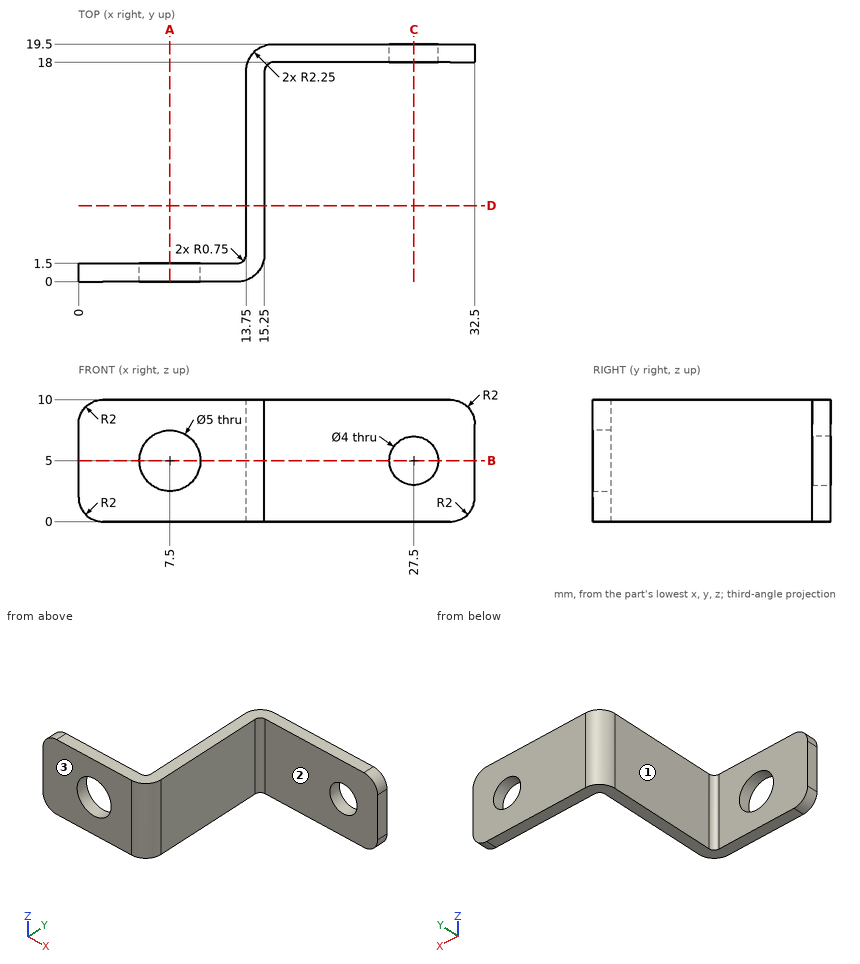
Geometry: see drawing. Coordinates: mm, zero at the bounding-box minimum. A direction names the side the tool comes from. Give positions to 0.01 mm unless a question says otherwise; leave off trailing zeros. Loops run counter-clockwise (first coordinate to the right, second up) from the corner with the lowest first, then second, coordinate; pieces in that order, holes last. Notation, with made-up numbers: (51, 88.25) - (91, 88.25) arc R23 cw to (91, 122.25) - close; hole circle Ø5 at (4.25, -37). An arc over 180 degrees is marked (long way). Use CSV: the item, a comma, the result in double quotes. Start each with the question number.
Item 1: Section B-B on z = 5. Return loops of the section in (x, y), then the cut area to 3 significant figures.
Item 2: Contact query for flat-ended pins moving along their axis: P1, Ø5, axis at y = 12, z = 9, coming from the +X side; P2, Ø4, axis at y = 10, z = 2, coming from the -X side; P3, Ø5, axis at x = 27, z = 4.5, coming from the -Y side. Output: stop coordinate, or through.
Item 3: Section A-A on x = 7.5. Return loops of the section in (y, z), then the cut area to 3 significant figures.
Item 4: Line query: line 1 (Y direction, x = 18, z = 4.25); line 2 (X direction, y = 12.5, z = 8); line 3 (X direction, y = 1.15, z = 5). Output: solid intervals per line, ascending.
Item 5: Section C-C on x = 27.5. Return loops of the section in (y, z), then the cut area to 3 significant figures.
Item 6: Reachability of the marked faces 1, 2 and 3 from +Z, -Z, +X, -X, +Y, -Y: full face, straight path, thin tool, end or side. Return the list, or none.
Item 7: Section D-D on y = 6.25. Return loops of the section in (x, z).
Ans:
1,outline,"(0, 0) - (5, 0) - (5, 1.5) - (0, 1.5) - close; (10, 0) - (13, 0) arc R2.25 ccw to (15.25, 2.25) - (15.25, 17.25) arc R0.75 cw to (16, 18) - (25.5, 18) - (25.5, 19.5) - (16, 19.5) arc R2.25 ccw to (13.75, 17.25) - (13.75, 2.25) arc R0.75 cw to (13, 1.5) - (10, 1.5) - close; (29.5, 18) - (32.5, 18) - (32.5, 19.5) - (29.5, 19.5) - close"
1,area,"60.3 mm2"
2,P1,"stops at x = 15.25"
2,P2,"stops at x = 13.75"
2,P3,"stops at y = 18"
3,outline,"(0, 0) - (1.5, 0) - (1.5, 2.5) - (0, 2.5) - close; (0, 7.5) - (1.5, 7.5) - (1.5, 10) - (0, 10) - close"
3,area,"7.50 mm2"
4,line 1,"y = 18 to 19.5"
4,line 2,"x = 13.75 to 15.25"
4,line 3,"x = 0 to 5, 10 to 14.96"
5,outline,"(18, 0) - (19.5, 0) - (19.5, 3) - (18, 3) - close; (18, 7) - (19.5, 7) - (19.5, 10) - (18, 10) - close"
5,area,"9.00 mm2"
6,face 1,"+Z, -Z, -X, +Y"
6,face 2,"+Z, -Z, +X, -Y"
6,face 3,"+Z, -Z, +X, -X, -Y"
7,outline,"(13.75, 0) - (15.25, 0) - (15.25, 10) - (13.75, 10) - close"
